Build history of the part. All positions in model axes, mm. A direction names the side the tool comes from. Round coordinates to 2 decimals unless told otherwise and drop trailing zeros. Loops run counter-clockwise (first coordinate to the right, second up) from the corner with the lowest first, then second, coordinate; pieces in that order, holes last. Notation, with made-up numbers: (60.5, 70) -> (91.5, 70) arc R33 ccw to (91.5, 102) -> close; hole circle Ø6 at (-32, -16). An arc over 180 degrees is marked (long way). Put each result on its own line as item: value. Start each with the question number.
Item 1: Drill centre lines: probe 1 along X at (y, z) = (-33.5, -4); probe 2 along X at (y, z) = (-114.5, -1.5); probe 3 along Z at (x, y) = (-9, -74). Where is each one in solid material? Low to high. Write a range as [from, to].
Item 2: Cut at B-B, the plane z = -1.75. List the corners of the cut face in (x, y).
Item 3: Flat gauge pins, fed straight in: pin 1 Ø1 at (y, z) = (-80.5, -5.5) entering from -X; pin 2 Ø4 at (y, z) = (-79.5, -4.5) entering from +X. Where does each tip first touch, or does it go through?
Item 4: Tool access for faces 1 (the flat face through (7.836, -73, -5)), 2 (the flat face through (-7.836, -73, -5)), 3 (the flat face through (0, 0, -2)): list every direction of +Z, -Z, +X, -X, +Y, -Y with a clear straight run to the whole face (end or side of a thin tool).
Item 5: Cut at C-C, the plane x = -9.5. List the corners of the cut face in (y, z), plus the area to 3 significant figures.
Item 6: Cut at A-A, the plane y = -138. List the corners of the cut face in (x, z), plus the area to 3 significant figures.
```python
from build123d import *

# Parameters (mm, degrees)
F0_W     = 9.4996
F0_H     = 2.7432
F1_DEPTH = 147.701


with BuildPart() as f1:
    # F0 (on Front) → F1 (new body)
    with BuildSketch(Plane.XZ):
        Polygon((9.4996, -1.3716), (0, -1.3716), (0, -6.5278), (7.8359, -6.5278), (7.8359, -3.0353), align=None)
        Polygon((0, -1.3716), (-9.4996, -1.3716), (-7.8359, -3.0353), (-7.8359, -6.5278), (0, -6.5278), align=None)
        with Locations((4.7498, 0)):
            Rectangle(F0_W, F0_H)
        Polygon((9.4996, 1.3716), (9.4996, -1.3716), (10.8712, 0), align=None)
        Polygon((0, 2.794), (0, 1.3716), (9.4996, 1.3716), (8.0772, 2.794), align=None)
        Polygon((-8.0772, 2.794), (-9.4996, 1.3716), (0, 1.3716), (0, 2.794), align=None)
        with Locations((-4.7498, 0)):
            Rectangle(F0_W, F0_H)
        Polygon((-10.8712, 0), (-9.4996, -1.3716), (-9.4996, 1.3716), align=None)
    extrude(amount=F1_DEPTH)


solid = f1.part
```
Reply:
1. probe 1: x = [-7.84, 7.84]
1. probe 2: x = [-9.37, 9.37]
1. probe 3: z = [-1.87, 1.87]
2. outline: (-9.12, -147.7) -> (9.12, -147.7) -> (9.12, 0) -> (-9.12, 0) -> close
3. pin 1: stops at x = -7.84
3. pin 2: stops at x = 8.37
4. face 1: -Z, +X, +Y, -Y
4. face 2: -Z, -X, +Y, -Y
4. face 3: +Z, -Z, +X, -X, +Y
5. outline: (-147.7, -1.37) -> (0, -1.37) -> (0, 1.37) -> (-147.7, 1.37) -> close
5. area: 405 mm^2
6. outline: (-10.87, 0) -> (-7.84, -3.04) -> (-7.84, -6.53) -> (7.84, -6.53) -> (7.84, -3.04) -> (10.87, 0) -> (8.08, 2.79) -> (-8.08, 2.79) -> close
6. area: 164 mm^2
